Geometry: final body of the model. Coordinates: model frame, mm. Face numbers are marked on the shaded views. A direction names the side the tool comes from. Give positions to 0.01 mm unless a question says otherwise; leave off trailing zeros. Write each loop counter-clockwise with the first axis right and the second up, starting at its lowest first coordinate (ties: lowest second). Pieces come first, ordered by that corner, then holes.
Q1. Cut plane C-C on z = 1.2. Return the cut outline in (x, y), plus the area to 3 significant figures.
Q2. Cut plane D-D on z = 3.55. Return the cut outline in (x, y), plus the area to 3 significant figures.
Q3. Cut plane A-A on y = 0. Return the cut outline in (x, z).
Q4. Reachability of the marked faces 1 and 2 from +Z, -Z, +X, -X, +Y, -Y: full face, straight path, thin tool, end or side. Return the list, or none.
Q5. Draft query along Y for the marked faces 3, 4 and 5. Return one class per face: pulls with the +Y half, pulls with the -Y half, needs draft (parallel to the pull), parting line crosses it, or undercut.
Q6. Line query: L1, parallel to Y at x = 0, z = 0.55; L2, parallel to Z at x = 5, y = 4.75; L3, parallel to Y at x = -2, z = 2.4. Output: solid intervals per line, ascending.
Q7. Pin query (flat end, axial travel): pin 1 (2 mm diameter, centred on x = 1, y = 7, fed in from -Z). Return the tip coordinate at first contact, or that it passes through.
```python
from build123d import *

# Parameters (mm, degrees)
F0_R     = 12.5
F0_R_2   = 11
F1_DEPTH = 4
F2_DEPTH = 2.6
F3_R     = 1


with BuildPart() as f1:
    # F0 (on Top) → F1 (new body)
    with BuildSketch(Plane.XY):
        Circle(F0_R)
        Circle(F0_R_2, mode=Mode.SUBTRACT)
        Circle(F0_R_2)
    extrude(amount=F1_DEPTH)

    # F0 (on Top) → F2 (cut)
    with BuildSketch(Plane.XY):
        Circle(F0_R_2)
    extrude(amount=F2_DEPTH, mode=Mode.SUBTRACT)

    # F3
    f3_edges = [f1.edges().sort_by_distance(p)[0] for p in [
        (-12.5, 0, 4),
    ]]
    fillet(f3_edges, radius=F3_R)


solid = f1.part
```
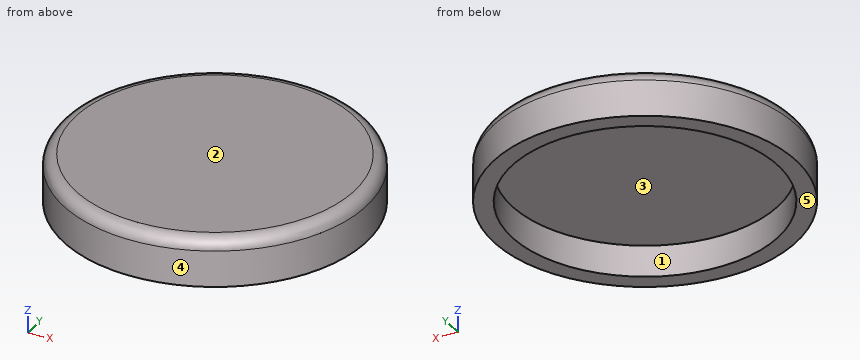
Data:
1. outline: circle Ø25 at (0, 0); hole circle Ø22 at (0, 0)
1. area: 111 mm2
2. outline: circle Ø24.67 at (0, 0)
2. area: 478 mm2
3. outline: (-12.5, 0) - (-11, 0) - (-11, 2.6) - (11, 2.6) - (11, 0) - (12.5, 0) - (12.5, 3) arc R1 ccw to (11.5, 4) - (-11.5, 4) arc R1 ccw to (-12.5, 3) - close
4. face 1: -Z
4. face 2: +Z, +X, -X, +Y, -Y
5. face 3: undercut
5. face 4: parting line crosses it
5. face 5: needs draft
6. L1: y = -12.5 to -11, 11 to 12.5
6. L2: z = 2.6 to 4
6. L3: y = -12.34 to -10.82, 10.82 to 12.34
7. pin 1: stops at z = 2.6
